Build history of the part. All positions in model axes, mm. A direction names the side the tool comes from. Give positions to 0.01 mm unless a question says otherwise; leave off trailing zeros. Order: outer loops, then holes, each group sorted by start corner. A loop starts at its lowest first (then second) coordinate and runs counter-clockwise, first axis right, second up. Notation, with made-up numbers: M 15.5,76.25 L 71.5,76.25 A14 ccw 71.5,97.25 Z; hole C 27.25,-11.5 d2. An arc over 180 degrees is marked long. One line per item, written item: value. Start each with the question number.
from build123d import *

# Parameters (mm, degrees)
SKETCH_1_R      = 1.4
SKETCH_1_R_2    = 2.1
EXTRUDE_1_DEPTH = 1


with BuildPart() as part:
    # 草图1 → 凸台-拉伸1 (new body)
    with BuildSketch(Plane.XY):
        with BuildLine():
            ThreePointArc((0, -3), (3, 0), (0, 3))
            ThreePointArc((0, 3), (-3, 6), (0, 9))
            ThreePointArc((0, 9), (8.949788871, -0.94935724), (-1.888121525, -8.79971574))
            ThreePointArc((-1.888121525, -8.79971574), (-5.13171085, -10.261262299), (-4.698844689, -13.792496777))
            ThreePointArc((-4.698844689, -13.792496777), (13.72027933, -19.725875002), (28.603853377, -7.358646923))
            ThreePointArc((28.603853377, -7.358646923), (28.557639821, -5.785568702), (27.387741629, -4.732929637))
            ThreePointArc((27.387741629, -4.732929637), (26.089784532, 4.065789705), (34, 0))
            ThreePointArc((34, 0), (20.055509911, -21.849807636), (-5.63484885, -18.404758393))
            ThreePointArc((-5.63484885, -18.404758393), (-8.201495332, -8.732960074), (0, -3))
        make_face()
        with Locations((0, 6)):
            Circle(SKETCH_1_R, mode=Mode.SUBTRACT)
        with Locations((0, -6)):
            Circle(SKETCH_1_R, mode=Mode.SUBTRACT)
        with Locations((29, 0)):
            Circle(SKETCH_1_R_2, mode=Mode.SUBTRACT)
    extrude(amount=EXTRUDE_1_DEPTH)


solid = part.part
1) Drill centre lines: line 1 (X direction, y = -6.5, z = 0.95); line 2 (Y direction, x = -0.5, z = 0.6); line 3 (X direction, y = 1, z = 0.2). Where is each one in solid material? Low to high.
2) Slice it at A-A (y = -6). List the corners of the cut face in (x, z), plus the area to 3 significant figures.
3) Slice it at D-D (x = 18). List the corners of the cut face in (y, z), plus the area to 3 significant figures.
4) Pull direction Y, two halves, no side cores. Call faces 1 (the flat face through (6, -4, 0)), 2 (the cylindrical face through (20.402, -21.686, 0.493)), 3 (the cylindrical face through (13.442, -19.778, 0.493)): pulls with the +Y half, pulls with the -Y half, needs draft (parallel to the pull), parting line crosses it, or undercut.
5) Slice it at C-C (y = 6). List the corners of the cut face in (x, z).
6) Slice it at B-B (z = 0.45). List the corners of the cut face in (x, y).
7) Tool access for faces 4 (the cylindrical face through (-8.25, -8.87, 0.49)), 5 (the cylindrical face through (28.57, -5.81, 0.49)): list every direction of +Z, -Z, +X, -X, +Y, -Y with a clear straight run to the whole face (end or side of a thin tool).
8) Drop flat-ended pins along their axis: P1, Ø3, axis at x = 0, y = -6, coming from the +Z side; P2, Ø1.7, axis at x = 0, y = 6, coming from the -Z side. Give the stop position or say it passes through.
Results list:
1. line 1: x = -6.99 to -1.31, 1.31 to 6.22, 28.74 to 33.11
1. line 2: y = -21.73 to -17.18, -8.99 to -7.31, -4.69 to -3.01, 3.04 to 4.69, 7.31 to 8.96
1. line 3: x = 2.83 to 8.94, 24.1 to 27.15, 30.85 to 33.9
2. outline: M -6.59,0 L -1.4,0 L -1.4,1 L -6.59,1 Z; M 1.4,0 L 6.71,0 L 6.71,1 L 1.4,1 Z; M 28.64,0 L 33.24,0 L 33.24,1 L 28.64,1 Z
2. area: 15.1 mm²
3. outline: M -22.69,0 L -18.39,0 L -18.39,1 L -22.69,1 Z
3. area: 4.30 mm²
4. face 1: needs draft
4. face 2: pulls with the -Y half
4. face 3: undercut
5. outline: M -3,0 L -1.4,0 L -1.4,1 L -3,1 Z; M 1.4,0 L 6.71,0 L 6.71,1 L 1.4,1 Z
6. outline: M -5.63,-18.4 A24.09 ccw 34,0 A5 ccw long 27.39,-4.73 A2 cw 28.6,-7.36 A20.09 cw -4.7,-13.79 A3 cw -1.89,-8.8 A9 ccw long 0,9 A3 ccw 0,3 A3 cw 0,-3 A8.73 ccw Z; hole C 0,-6 d2.8; hole C 0,6 d2.8; hole C 29,0 d4.2
7. face 4: +Z, -Z, -X
7. face 5: +Z, -Z
8. P1: stops at z = 1
8. P2: passes through
